Geometry: final body of the model. Coordinates: model frame, mm. Face numbers are marked on the shaded views. A direction names the side the tool comes from. Round coordinates to 2 decimals unless told otherwise and drop trailing zeros. Loops run counter-clockwise (first coordinate to the right, second up) from the corner with the lowest first, then second, coordinate; pieces in that order, holes last. Notation, with made-up numbers: M 76,25.5 L 90,25.5 A18 ccw 90,30.5 Z; hole C 60,66 d11. An arc over 180 degrees is marked long. Return JSON: item names as keys, results as strings.
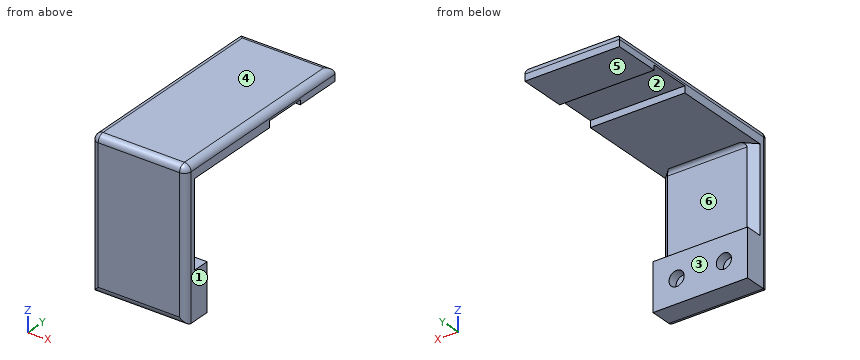
from build123d import *

# Parameters (mm, degrees)
F1_DEPTH = 50
F2_R     = 3.5
F3_R     = 3.5
F4_R     = 4
F5_DEPTH = 5
F6_SIZE  = 4
F7_R     = 2


with BuildPart() as f1:
    # F0 (on Right) → F1 (new body)
    with BuildSketch(Plane.YZ):
        Polygon((97, 8), (-10, 8), (-10, -70), (5, -70), (5, -45), (0, -45), (0, 0), (50, 0), (50, 3.5), (72, 3.5), (72, 1), (97, 1), align=None)
    extrude(amount=F1_DEPTH)

    # F2
    f2_edges = [f1.edges().sort_by_distance(p)[0] for p in [
        (25, -10, 8),
    ]]
    fillet(f2_edges, radius=F2_R)

    # F3
    f3_edges = [f1.edges().sort_by_distance(p)[0] for p in [
        (50, 45.25, 8),
        (25, 97, 8),
        (0, 45.25, 8),
        (25, -10, -70),
    ]]
    fillet(f3_edges, radius=F3_R)

    # F4 (on face) → F5 (cut)
    with BuildSketch(Plane(origin=(0, 5, 0), x_dir=(-1, 0, 0), z_dir=(0, 1, 0))):
        with Locations((-37.5, -57.5)):
            Circle(F4_R)
        with Locations((-12.5, -57.5)):
            Circle(F4_R)
    extrude(amount=-F5_DEPTH, mode=Mode.SUBTRACT)

    # F6
    f6_edges = [f1.edges().sort_by_distance(p)[0] for p in [
        (50, 0, -22.5),
        (0, 0, -22.5),
    ]]
    chamfer(f6_edges, length=F6_SIZE)

    # F7
    f7_edges = [f1.edges().sort_by_distance(p)[0] for p in [
        (25, 0, 0),
    ]]
    fillet(f7_edges, radius=F7_R)


solid = f1.part
Q1. Reachability of the marked faces 1 and 2 from +Z, -Z, +X, -X, +Y, -Y: full face, straight path, thin tool, end or side. Return the list, or none.
Determined:
{"face 1": "+Z, -Z, +X, +Y, -Y", "face 2": "-Z, +X, -X"}
Q2. Section query B-B (x = 29.5). Output: boundary loops of the cut face in (y, z), plus the area to 3 significant figures.
Determined:
{"outline": "M -10,-66.5 A3.5 ccw -6.5,-70 L 5,-70 L 5,-45 L 0,-45 L 0,-2 A2 cw 2,0 L 50,0 L 50,3.5 L 72,3.5 L 72,1 L 97,1 L 97,4.5 A3.5 ccw 93.5,8 L -6.5,8 A3.5 ccw -10,4.5 Z", "area": "1,570 mm^2"}
Q3. Material intervals for L1, parallel to Z at x = 37.5, y = 3; L2, parallel to Z at x = 12, y = 1; L3, parallel to Z at x = 23.5, y = 28.5, sorted ascending.
Determined:
{"L1": "z = -70 to -61.5, -53.5 to -45, 0 to 8", "L2": "z = -70 to -61.47, -53.53 to -45, -0.27 to 8", "L3": "z = 0 to 8"}
Q4. Section query C-C (z = -12). Output: boundary loops of the cut face in (x, y), plus the area to 3 significant figures.
Determined:
{"outline": "M 0,-6.5 A3.5 ccw 3.5,-10 L 46.5,-10 A3.5 ccw 50,-6.5 L 50,-4 L 46,0 L 4,0 L 0,-4 Z", "area": "479 mm^2"}
Q5. Section query A-A (y = 36). Output: boundary loops of the cut face in (x, z).
Determined:
{"outline": "M 0,0 L 50,0 L 50,4.5 A3.5 ccw 46.5,8 L 3.5,8 A3.5 ccw 0,4.5 Z"}
Q6. Section query D-D (y = 70). Output: boundary loops of the cut face in (x, z), plus the area to 3 significant figures.
Determined:
{"outline": "M 0,3.5 L 50,3.5 L 50,4.5 A3.5 ccw 46.5,8 L 3.5,8 A3.5 ccw 0,4.5 Z", "area": "220 mm^2"}
Q7. Pull-direction query (Z, two-part tool) for the marked faces 3, 4, 5 and 6; classes: pulls with the +Z half, pulls with the -Z half, needs draft (parallel to the pull), parting line crosses it, or undercut.
Determined:
{"face 3": "needs draft", "face 4": "pulls with the +Z half", "face 5": "pulls with the -Z half", "face 6": "undercut"}
Q8. Pin query (flat end, axial travel): pin 1 (9 mm diameter, centred on x = 37.5, z = -57.5, fed in from +Y); pin 2 (15 mm diameter, centred on x = 18, y = 23.5, fed in from -Z); pin 3 (11 mm diameter, centred on x = 33, y = 61, fed in from -Z); pin 4 (10 mm diameter, centred on y = 47.5, z = -6.5, fed in from -X). Return the tip coordinate at first contact, or that it passes through.
Determined:
{"pin 1": "stops at y = 5", "pin 2": "stops at z = 0", "pin 3": "stops at z = 3.5", "pin 4": "passes through"}
